Read the model definition and answer for the solid it produces. Units are mm, in the model's axes. Give positions to 0.01 mm unless a question says otherwise; leave off trailing zeros. Write each loop counter-clockwise with the first axis right and the second up, starting at its lowest first coordinate (ties: lowest second). Pieces come first, ordered by that corner, then holes. Notation, with made-up numbers: (19.5, 19.5) - (33.5, 19.5) arc R30 ccw to (33.5, 55.5) - close; hole circle Ø2 at (67.25, -15). An arc over 180 degrees is marked (long way). Answer as a JSON object with one key per item and string values. Group by question number.
```python
from build123d import *

# Parameters (mm, degrees)
F0_R     = 21.913418
F0_R_2   = 25.159395
F1_DEPTH = 3


with BuildPart() as f1:
    # F0 (on Front) → F1 (new body)
    with BuildSketch(Plane.XZ):
        Polygon((-68.047404, 49.813341), (-70.425756, 49.813341), (-70.425756, -54.305792), (64.876266, -54.305792), (64.876266, 49.549077), align=None)
        with Locations((-41.092701, 0)):
            Circle(F0_R, mode=Mode.SUBTRACT)
        with Locations((29.993711, 0)):
            Circle(F0_R_2, mode=Mode.SUBTRACT)
    extrude(amount=-F1_DEPTH)


solid = f1.part
```
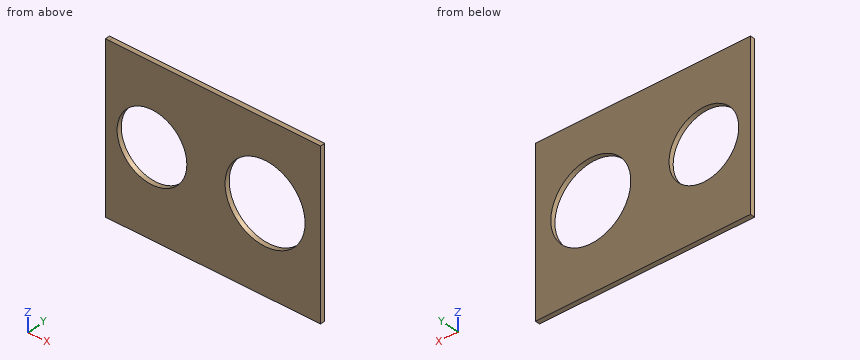
1) Find section D-D, the plane z = 14. Write down the section's boundary in (x, y), and give its area (3 significant figures).
2) A flat-ended cylindrical pin translates along its axis: pin 1 Ø1 at (x, z) = (32.5, 33.5) entering from -Y. Find the tip coordinate at first contact, or state that the pin passes through.
3) Find section B-B, the plane y = 0.55. Write down the section's boundary in (x, z).
4) Find section C-C, the plane x = -29. Write down the section's boundary in (y, z), and give its area (3 significant figures).
5) Find section A-A, the plane z = 0. Write down the section's boundary in (x, y), and give its area (3 significant figures).
6) Find the intervals of material crossed by line 1 (X direction, y = 1.25, z = -10); line 2 (X direction, y = 2.85, z = 7); line 3 (Z direction, x = 26.5, y = 0.45), in increasing order. Write a range as [from, to].
Values follow:
{
 "1": {"outline": "(-70.43, 0) - (-57.95, 0) - (-57.95, 3) - (-70.43, 3) - close; (-24.23, 0) - (9.09, 0) - (9.09, 3) - (-24.23, 3) - close; (50.9, 0) - (64.88, 0) - (64.88, 3) - (50.9, 3) - close", "area": "179 mm2"},
 "2": {"pin 1": "stops at y = 0"},
 "3": {"outline": "(-70.43, -54.31) - (64.88, -54.31) - (64.88, 49.55) - (-68.05, 49.81) - (-70.43, 49.81) - close; hole circle Ø43.83 at (-41.09, 0); hole circle Ø50.32 at (29.99, 0)"},
 "4": {"outline": "(0, -54.31) - (3, -54.31) - (3, -18.27) - (0, -18.27) - close; (0, 18.27) - (3, 18.27) - (3, 49.74) - (0, 49.74) - close", "area": "202 mm2"},
 "5": {"outline": "(-70.43, 0) - (-63.01, 0) - (-63.01, 3) - (-70.43, 3) - close; (-19.18, 0) - (4.83, 0) - (4.83, 3) - (-19.18, 3) - close; (55.15, 0) - (64.88, 0) - (64.88, 3) - (55.15, 3) - close", "area": "123 mm2"},
 "6": {"line 1": "x = [-70.43, -60.59], [-21.59, 6.91], [53.08, 64.88]", "line 2": "x = [-70.43, -61.86], [-20.33, 5.83], [54.16, 64.88]", "line 3": "z = [-54.31, -24.92], [24.92, 49.63]"}
}
